Geometry check sheet. Reference: drawing and pictorial views, mm from the part's lowest x, y, z. Give positions to 0.01 mm unless a question says otherwise; leave off trailing zeros. Write each loop counter-clockwise with the first axis right and the second up, starting at its lowest first coordinate (ties: lowest second). Pieces come first, ordered by that corner, then holes. Notation, with made-up numbers: (86, 80.25) -> (99, 80.25) arc R12 cw to (99, 87.25) -> close; hole circle Ø2 at (60.5, 47). An arc over 180 degrees is marked (long way). Answer as CSV lines item,"result".
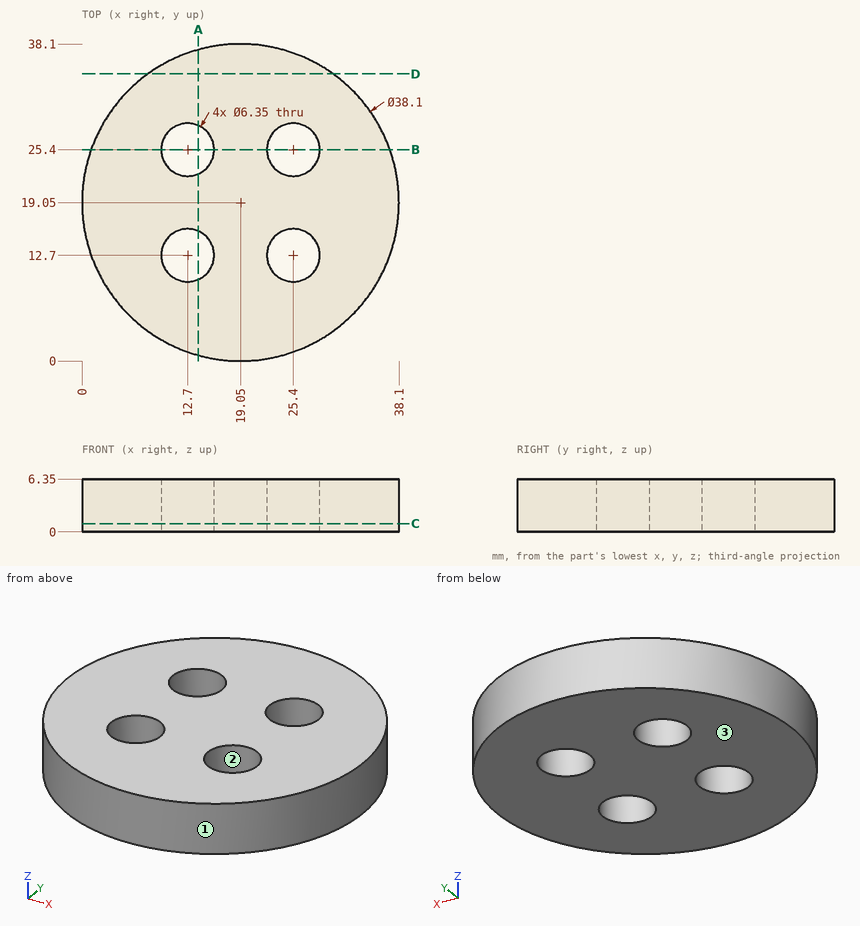
1) Draft check along Y on the marked faces 1, 2 and 3. Enter one of: +Y half, -Y half, draft (parallel to the pull), parting line (faces both ways), or undercut.
Reported:
face 1,"parting line"
face 2,"undercut"
face 3,"draft"
2) Section check A-A (x = 14). Record the boundary of the cut face in (y, z).
Reported:
outline,"(0.68, 0) -> (9.8, 0) -> (9.8, 6.35) -> (0.68, 6.35) -> close; (15.6, 0) -> (22.5, 0) -> (22.5, 6.35) -> (15.6, 6.35) -> close; (28.3, 0) -> (37.42, 0) -> (37.42, 6.35) -> (28.3, 6.35) -> close"
3) Section check D-D (y = 34.5). Record the boundary of the cut face in (x, z).
Reported:
outline,"(7.91, 0) -> (30.19, 0) -> (30.19, 6.35) -> (7.91, 6.35) -> close"
4) Depth check by flat-ended pin: pin 1 (2 mm diameter, centred on y = 14.5, z = 3, fed in from -X); pin 2 (1 mm diameter, centred on x = 31.5, z = 3, fed in from +Y); pin 3 (4 mm diameter, centred on x = 25.4, y = 25.4, fed in from -Z); pin 4 (10 mm diameter, centred on x = 12.7, y = 25.4, fed in from +Z). Enter the tip coordinate at first touch or a pass-through.
Reported:
pin 1,"x = 0.33"
pin 2,"y = 33.89"
pin 3,"through"
pin 4,"z = 6.35"
5) Scan lines: line 1 along X through (y, z) = (15, 1.75); line 2 along Y through (x, z) = (25.4, 2.5) (3 decimals); line 3 along X through (y, z) = (14, 3.5). Record each from-to range of solid material in increasing order.
Reported:
line 1,"0.44 to 10.51, 14.89 to 23.21, 27.59 to 37.66"
line 2,"1.089 to 9.525, 15.875 to 22.225, 28.575 to 37.011"
line 3,"0.68 to 9.8, 15.6 to 22.5, 28.3 to 37.42"
6) Section check B-B (y = 25.4). Record the boundary of the cut face in (x, z) (3 decimals), and give its area (3 significant figures).
Reported:
outline,"(1.089, 0) -> (9.525, 0) -> (9.525, 6.35) -> (1.089, 6.35) -> close; (15.875, 0) -> (22.225, 0) -> (22.225, 6.35) -> (15.875, 6.35) -> close; (28.575, 0) -> (37.011, 0) -> (37.011, 6.35) -> (28.575, 6.35) -> close"
area,"147 mm²"
7) Section check C-C (z = 1). Record the boundary of the cut face in (x, y) (3 decimals), and give its area (3 significant figures).
Reported:
outline,"circle Ø38.1 at (19.05, 19.05); hole circle Ø6.35 at (12.7, 12.7); hole circle Ø6.35 at (12.7, 25.4); hole circle Ø6.35 at (25.4, 12.7); hole circle Ø6.35 at (25.4, 25.4)"
area,"1,010 mm²"
